from build123d import *

# Parameters (mm, degrees)
CROQUIS1_W              = 100
CROQUIS1_H              = 10
SALIENTE_EXTRUIR1_DEPTH = 5
CROQUIS2_W              = 5
CROQUIS2_H              = 10
SALIENTE_EXTRUIR2_DEPTH = 15
CROQUIS3_R              = 0.8
CORTAR_EXTRUIR1_DEPTH   = 5
CROQUIS4_W              = 5.029184128
CROQUIS4_H              = 10
SALIENTE_EXTRUIR3_DEPTH = 27
CROQUIS5_R              = 0.8
CORTAR_EXTRUIR2_DEPTH   = 10


with BuildPart() as part:
    # Croquis1 → Saliente-Extruir1 (new body)
    with BuildSketch(Plane(origin=(0, 0, 0), x_dir=(1, 0, 0), z_dir=(0, 1, 0))):
        Rectangle(CROQUIS1_W, CROQUIS1_H)
    extrude(amount=SALIENTE_EXTRUIR1_DEPTH)

    # Croquis2 → Saliente-Extruir2 (add)
    with BuildSketch(Plane(origin=(0, 5, 0), x_dir=(1, 0, 0), z_dir=(0, 1, 0))):
        with Locations((-47.5, 0)):
            Rectangle(CROQUIS2_W, CROQUIS2_H)
        with Locations((47.5, 0)):
            Rectangle(CROQUIS2_W, CROQUIS2_H)
    extrude(amount=SALIENTE_EXTRUIR2_DEPTH)

    # Croquis3 → Cortar-Extruir1 (cut)
    with BuildSketch(Plane(origin=(0, 20, 0), x_dir=(1, 0, 0), z_dir=(0, 1, 0))):
        with Locations((-47.5, 0)):
            Circle(CROQUIS3_R)
        with Locations((47.5, 0)):
            Circle(CROQUIS3_R)
    extrude(amount=-CORTAR_EXTRUIR1_DEPTH, mode=Mode.SUBTRACT)

    # Croquis4 → Saliente-Extruir3 (add)
    with BuildSketch(Plane.XZ):
        Rectangle(CROQUIS4_W, CROQUIS4_H)
    extrude(amount=SALIENTE_EXTRUIR3_DEPTH)

    # Croquis5 → Cortar-Extruir2 (cut)
    with BuildSketch(Plane.XZ.offset(27)):
        Circle(CROQUIS5_R)
    extrude(amount=-CORTAR_EXTRUIR2_DEPTH, mode=Mode.SUBTRACT)


solid = part.part
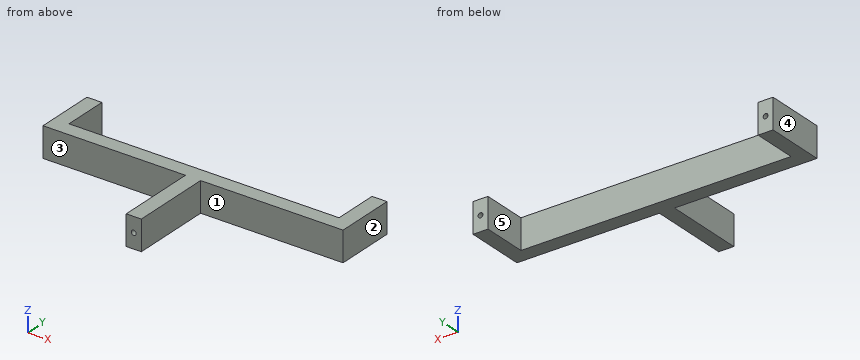
Source: CAD feature listing. Evaluate the final solid. Frame: model axes, mm. Face numbers are marked on the shaded views. A direction names the side the tool comes from. Give positions to 0.01 mm unless a question says otherwise; leave off trailing zeros. Write each loop counter-clockwise with the first axis right and the second up, starting at its lowest first coordinate (ties: lowest second). Pieces come first, ordered by that corner, then holes. Notation, with made-up numbers: M 28.5,-24 L 66.5,-24 A13 cw 66.5,-14 Z; hole C 3,65.5 d2. An arc over 180 degrees is marked long. Return JSON: item names as keys, results as strings. Group by question number.
1) Pin query (flat end, axial travel): P1, Ø2, axis at x = 0, z = 0, coming from the -Y side; P2, Ø5, axis at x = -21.5, z = 1, coming from the +Y side; P3, Ø1.8, axis at x = -47.5, z = 0, coming from the -Y side; P4, Ø5, axis at y = -20, z = -2, coming from the -X side. Return the tip coordinate at first contact, or that it passes through.
2) Set-up query: the marked faces 1, 2, 3, 4 and 5. Return all of +Z, -Z, +X, -X, +Y, -Y with unobstructed straight access to the full face (end or side cutting, diameter ignored); none if empty.
3) Cut plane D-D, the plane y = -13.5. Output: boundary loops of the cut face in (x, z), plus the area to 3 significant figures.
4) Cut plane B-B, the plane y = -19.5. Output: boundary loops of the cut face in (x, z).
5) Cut plane C-C, the plane x = -34. Output: boundary loops of the cut face in (y, z).
6) Cut plane A-A, the plane z = 3.5. Output: boundary loops of the cut face in (x, y).
7) Material intervals for line 1 along Z through (x, y) = (0, -19.5); line 2 along X through (y, z) = (12.5, 3.75); line 3 along X through (y, z) = (-18.5, -1.75), sorted ascending. Write a range as [from, to].
Recorded:
{
 "1": {"P1": "stops at y = -27", "P2": "stops at y = 5", "P3": "stops at y = 0", "P4": "stops at x = -2.51"},
 "2": {"face 1": "+Z, -Z, +X, -Y", "face 2": "+Z, -Z, +X, +Y, -Y", "face 3": "+Z, -Z, -X, -Y", "face 4": "+Z, -Z, -X, +Y, -Y", "face 5": "+Z, -Z, +Y"},
 "3": {"outline": "M -2.51,-5 L 2.51,-5 L 2.51,5 L -2.51,5 Z", "area": "50.3 mm²"},
 "4": {"outline": "M -2.51,-5 L 2.51,-5 L 2.51,5 L -2.51,5 Z; hole C 0,0 d1.6"},
 "5": {"outline": "M 0,-5 L 5,-5 L 5,5 L 0,5 Z"},
 "6": {"outline": "M -50,0 L -2.51,0 L -2.51,-27 L 2.51,-27 L 2.51,0 L 50,0 L 50,20 L 45,20 L 45,5 L -45,5 L -45,20 L -50,20 Z"},
 "7": {"line 1": "z = [-5, -0.8], [0.8, 5]", "line 2": "x = [-50, -45], [45, 50]", "line 3": "x = [-2.51, 2.51]"}
}
